Check sheet for the modelled part. Datum: model origin and axes. Units: mm. A direction names the side the tool comes from. Give positions to 0.01 mm unless a question says otherwise; leave off trailing zeros. Write each loop counter-clockwise with the first axis right and the second up, starting at its lowest first coordinate (ties: lowest second). Pieces come first, ordered by that corner, then holes. Notation, with made-up numbers: (21.25, 18.5) -> (28.25, 18.5) arc R27 cw to (28.25, 50.5) -> close; hole circle Ø5 at (-29.75, -20). An arc over 180 degrees is marked (long way). Return JSON: item names as keys, results as strings.
from build123d import *

# Parameters (mm, degrees)
F0_R     = 50
F0_R_2   = 30
F1_DEPTH = 160
F3_START = 30
F2_R     = 40
F3_DEPTH = 50
F4_R     = 10
F6_DEPTH = 17.5
F7_R     = 10
F8_R     = 4.99999
F9_R     = 5


# Not quite as in the source:
# - a fillet or chamfer is up to 0.001 mm smaller than in the source, because OpenCascade refuses the exact size


with BuildPart() as f1:
    # F0 (on Right) → F1 (new body)
    with BuildSketch(Plane.YZ):
        Circle(F0_R)
        Circle(F0_R_2, mode=Mode.SUBTRACT)
    extrude(amount=F1_DEPTH)

    # F2 (on Front) → F3 (join)
    with BuildSketch(Plane.XZ.offset(F3_START)):
        with Locations((80, 0)):
            Circle(F2_R)
    extrude(amount=F3_DEPTH)

    # F4
    f4_edges = [f1.edges().sort_by_distance(p)[0] for p in [
        (40, -80, 0),
    ]]
    fillet(f4_edges, radius=F4_R)

    # F5 (on Top) → F6 (join, symmetric)
    with BuildSketch(Plane.XY):
        Polygon((135, -80), (110, -80), (65, -80), (65, -100), (135, -100), (173.0335205793, -134.9323159456), (323.0335205793, -134.9323159456), (323.0335205793, -124.9323159456), (176.2279570103, -124.9323159456), align=None)
    extrude(amount=F6_DEPTH, both=True)

    # F7
    f7_edges = [f1.edges().sort_by_distance(p)[0] for p in [
        (65, -90, -17.5),
        (65, -90, 17.5),
        (323.033521, -129.932316, -17.5),
        (323.033521, -129.932316, 17.5),
    ]]
    fillet(f7_edges, radius=F7_R)

    # F8 (radius 5 in the source; OpenCascade refuses exactly that, so slightly less here)
    f8_edges = [f1.edges().sort_by_distance(p)[0] for p in [
        (243.033521, -134.932316, -17.5),
        (244.630739, -124.932316, -17.5),
    ]]
    fillet(f8_edges, radius=F8_R)

    # F9
    f9_edges = [f1.edges().sort_by_distance(p)[0] for p in [
        (160, -50, 0),
        (0, -50, 0),
    ]]
    fillet(f9_edges, radius=F9_R)


solid = f1.part
(1) Set-up check for faces 4 (the flat face through (123, -97, 17.5)), 5 (the flat face through (123, -97, -17.5)), 6 (the cylindrical face through (98.458, -54.163, -35.487)), 7 (the flat face through (160, 29, -9)): record each of +Z, -Z, +X, -X, +Y, -Y from which the full face is reachable in a straight line by a thin tool's end or side.
Reply:
{"face 4": "+Z, +X, -X, -Y", "face 5": "-Z, +X, -X, -Y", "face 6": "none", "face 7": "+Z, -Z, +X, +Y"}
(2) Cross-section at A-A on y = 0. Enter the section's corners in (x, z).
Reply:
{"outline": "(0, -45) arc R5 ccw to (5, -50) -> (155, -50) arc R5 ccw to (160, -45) -> (160, -30) -> (0, -30) -> close; (0, 30) -> (160, 30) -> (160, 45) arc R5 ccw to (155, 50) -> (5, 50) arc R5 ccw to (0, 45) -> close"}
(3) Cross-section at C-C on x = 80. Enter the section's corners in (y, z).
Reply:
{"outline": "(-100, -17.5) -> (-80, -17.5) -> (-80, -30) arc R10 ccw to (-70, -40) -> (-30, -40) arc R50 ccw (long way) to (-30, 40) -> (-70, 40) arc R10 ccw to (-80, 30) -> (-80, 17.5) -> (-100, 17.5) -> close; hole circle Ø60 at (0, 0)"}
(4) Thickness scan on L1, parallel to Y at x = 34, z = 0.5; L2, parallel to Z at x = 36, y = -2. Record the ranges inside material, lowest first.
Reply:
{"L1": "-50 to -30, 30 to 50", "L2": "-49.96 to -29.93, 29.93 to 49.96"}
(5) Depth check by flat-ended pin: pin 1 Ø1.5 at (x, y) = (132, -31) entering from -Z; pin 2 Ø17.5 at (x, z) = (109, 1.5) entering from -Y; pin 3 Ø12 at (y, z) = (-90, 3) entering from -X; pin 4 Ø1.5 at (y, z) = (-28.5, -6) entering from +X. Enter the tip coordinate at first touch or a pass-through.
Reply:
{"pin 1": "z = -39.81", "pin 2": "y = -100", "pin 3": "x = 65", "pin 4": "through"}
(6) Release check for a two-part mould opening along Y. For faces 1 (the flat face through (0, 29, -9)), 2 (the flat face through (153.14, -99.77, 0.25)), 3 (the flat face through (100, -100, 0)) record: pulls with the +Y half, pulls with the -Y half, needs draft (parallel to the pull), parting line crosses it, or undercut.
Reply:
{"face 1": "needs draft", "face 2": "undercut", "face 3": "pulls with the -Y half"}
